```python
from build123d import *

# Parameters (mm, degrees)
ESQUISSE1_R        = 1.6
BOSS_EXTRU_1_DEPTH = 1


with BuildPart() as part:
    # Esquisse1 → Boss.-Extru.1 (new body)
    with BuildSketch(Plane(origin=(0, 0, 0), x_dir=(1, 0, 0), z_dir=(0, 1, 0))):
        Polygon((0, 0), (0, 255), (55, 255), (55, 55), (58, 55), (58, 8.2), (55, 8.2), (31.2, 8.2), (31.2, 0), align=None)
        with Locations(Location((46, 60, 0), (0, 0, 270))):
            Circle(ESQUISSE1_R, mode=Mode.SUBTRACT)
        with Locations(Location((46, 120, 0), (0, 0, 270))):
            Circle(ESQUISSE1_R, mode=Mode.SUBTRACT)
        with Locations(Location((46, 180, 0), (0, 0, 270))):
            Circle(ESQUISSE1_R, mode=Mode.SUBTRACT)
        with Locations(Location((46, 240, 0), (0, 0, 270))):
            Circle(ESQUISSE1_R, mode=Mode.SUBTRACT)
    extrude(amount=BOSS_EXTRU_1_DEPTH)


solid = part.part
```
CAD build for the part. Positions are in the model's coordinates, mm. Give positions to 0.01 mm unless a question says otherwise; leave off trailing zeros. Order: outer loops, then holes, each group sorted by start corner. A loop starts at its lowest first (then second) coordinate and runs counter-clockwise, first axis right, second up.
(1) Saw through at A-A, the plane y = 0.2. Give the cut face in (x, z).
(2) Drill centre lines: L1, parallel to X at y = 0.45, z = -60; L2, parallel to Z at x = 43.5, y = 0.35; L3, parallel to X at y = 0.45, z = -104.5. Where is each one in solid material? Low to high.
(3) Flat gauge pins, fed straight in: pin 1 (0.5 mm diameter, centred on y = 0.5, z = -160, fed in from +X); pin 2 (0.5 mm diameter, centred on y = 0.5, z = -4, fed in from +X). Where does each tip first touch, or does it go through?
(4) Saw through at B-B, the plane x = 41. Give the cut face in (y, z), then the cut area to 3 significant figures.
Results found:
1. outline: (0, -255) - (55, -255) - (55, -55) - (58, -55) - (58, -8.2) - (31.2, -8.2) - (31.2, 0) - (0, 0) - close; hole circle Ø3.2 at (46, -240); hole circle Ø3.2 at (46, -180); hole circle Ø3.2 at (46, -120); hole circle Ø3.2 at (46, -60)
2. L1: x = 0 to 44.4, 47.6 to 55
2. L2: z = -255 to -8.2
2. L3: x = 0 to 55
3. pin 1: stops at x = 55
3. pin 2: stops at x = 31.2
4. outline: (0, -255) - (1, -255) - (1, -8.2) - (0, -8.2) - close
4. area: 247 mm2
